from build123d import *

# Parameters (mm, degrees)
F1_DEPTH = 13.9
F2_R     = 5
F3_R     = 5
F4_R     = 5
F5_SIZE  = 1


with BuildPart() as f1:
    # F0 (on Top) → F1 (new body)
    with BuildSketch(Plane.XY):
        with BuildLine():
            Line((-18.716553, -5.452939), (-18.716553, -65.452939))
            Line((-18.716553, -65.452939), (-13.716553, -65.452939))
            Line((-13.716553, -65.452939), (-13.716553, -7.784481))
            Line((-13.716553, -7.784481), (54.288781, 49.278771))
            ThreePointArc((54.288781, 49.278771), (57.086409, 56.09465), (63.865801, 58.979571))
            Line((63.865801, 58.979571), (58.071121, 58.979571))
            Line((58.071121, 58.979571), (-18.716553, -5.452939))
        make_face()
        with BuildLine():
            Line((64.114961, 58.979571), (63.865801, 58.979571))
            ThreePointArc((63.865801, 58.979571), (57.086409, 56.09465), (54.288781, 49.278771))
            Line((54.288781, 49.278771), (54.288781, 46.61191))
            ThreePointArc((54.288781, 46.61191), (63.988781, 36.498362), (73.688781, 46.61191))
            Line((73.688781, 46.61191), (73.688781, 49.52791))
            ThreePointArc((73.688781, 49.52791), (70.80626, 56.182743), (64.114961, 58.979571))
        make_face()
        with BuildLine():
            Line((56.688781, 49.52791), (71.288781, 49.52791))
            Line((71.288781, 49.52791), (71.288781, 46.61191))
            Line((71.288781, 46.61191), (72.188781, 46.61191))
            ThreePointArc((72.188781, 46.61191), (63.988781, 37.996817), (55.788781, 46.61191))
            Line((55.788781, 46.61191), (56.688781, 46.61191))
            Line((56.688781, 46.61191), (56.688781, 49.52791))
        make_face(mode=Mode.SUBTRACT)
        with BuildLine():
            ThreePointArc((64.114961, 58.979571), (63.990381, 58.98037), (63.865801, 58.979571))
            Line((63.865801, 58.979571), (64.114961, 58.979571))
        make_face()
    extrude(amount=F1_DEPTH)

    # F2
    f2_edges = [f1.edges().sort_by_distance(p)[0] for p in [
        (58.071121, 58.979571, 6.95),
    ]]
    fillet(f2_edges, radius=F2_R)

    # F3
    f3_edges = [f1.edges().sort_by_distance(p)[0] for p in [
        (54.288781, 49.278771, 6.95),
    ]]
    fillet(f3_edges, radius=F3_R)

    # F4
    f4_edges = [f1.edges().sort_by_distance(p)[0] for p in [
        (-13.716553, -7.784481, 6.95),
        (-18.716553, -5.452939, 6.95),
    ]]
    fillet(f4_edges, radius=F4_R)

    # F5
    f5_edges = [f1.edges().sort_by_distance(p)[0] for p in [
        (-18.716553, -65.452939, 6.95),
        (-16.216553, -65.452939, 13.9),
        (-13.716553, -65.452939, 6.95),
        (-16.216553, -65.452939, 0),
    ]]
    chamfer(f5_edges, length=F5_SIZE)


solid = f1.part
Can you work these out from the model? Positions are in its coordinate system, mm. A direction names the side the tool comes from. Coordinates: 2 decimals unless noted, no trailing zeros. Write each loop counter-clockwise with the first axis right and the second up, starting at its lowest first coordinate (ties: lowest second). Pieces come first, ordered by that corner, then holes. Notation, with made-up numbers: (-26.5, -23) -> (-8.5, -23) arc R15 cw to (-8.5, 4) -> close; hole circle Ø3 at (37.25, 31.25). An arc over 180 degrees is marked (long way). Write each question's results on one line, items separated by ' | '. Start each with the question number.
Item 1: On a 3-axis mill with a long thin cutter (end or side, diameter ignored), from which of +Z, -Z, +X, -X, +Y, -Y can I reach the whole of each face in a straight line? I mean faces 1 (the flat face through (-18.717, -36, 7)), 2 (the flat face through (-13.717, -38, 7)), 3 (the flat face through (71.289, 48, 7)). Say none if no direction works.
Item 2: If we section it at B-B, the plane x = 25.5: Write out the boundary of the cut face in (y, z), and give its area (3 significant figures).
Item 3: Thinking about a two-plate mould opening in Y: for faces 4 (the cylindrical face through (-13.235, -7.975, 7.047)), 5 (the cylindrical face through (70.88, 56.11, 6.85)), 6 (the cylindrical face through (64.2, 38, 6.9)), 7 (the flat face through (64, 49.528, 7)), which applies, released by +Y, released by -Y, zero draft, split by the parting line, or undercut?
Item 4: Please list where these lines run through material, in increasing order: probe 1 along X at (y, z) = (39, 7.25); probe 2 along X at (y, z) = (-60, 4.75); probe 3 along X at (y, z) = (41, 13).
Item 5: If we section it at A-A, the plane y = -13.5: Write out the boundary of the cut face in (x, z).
Item 6: I'm going to push flat-ended pins straight in: P1, Ø2.5, axis at y = 48, z = 7, coming from the -X side; P2, Ø8, axis at y = -19, z = 8, coming from the +X side; P3, Ø7, axis at x = 60.5, z = 6.5, coming from the -Y side. Where does each tip first touch, or does it pass through?
Answer block:
1) face 1: +Z, -Z, -X, +Y, -Y | face 2: +Z, -Z, +X, -Y | face 3: +Z, -Z
2) outline: (25.12, 0) -> (31.65, 0) -> (31.65, 13.9) -> (25.12, 13.9) -> close | area: 90.7 mm²
3) face 4: released by -Y | face 5: released by +Y | face 6: undercut | face 7: undercut
4) probe 1: 34.26 to 42.04, 57.48 to 60.06, 67.92 to 70.49 | probe 2: -18.72 to -13.72 | probe 3: 36.64 to 44.42, 55.79 to 57.64, 70.34 to 72.18
5) outline: (-18.72, 0) -> (-13.72, 0) -> (-13.72, 13.9) -> (-18.72, 13.9) -> close
6) P1: x = 43.5 | P2: x = -13.72 | P3: y = 36.5
